from build123d import *

# Parameters (mm, degrees)
SKETCH_1_R          = 30
EXTRUDE_1_DEPTH     = 1
SKETCH_2_R          = 49
EXTRUDE_2_DEPTH     = 8
SKETCH_3_R          = 31
EXTRUDE_3_DEPTH     = 10
SKETCH_4_R          = 25
CUT_EXTRUDE_1_DEPTH = 1
SKETCH_5_R          = 15.5
CUT_EXTRUDE_2_DEPTH = 6
SKETCH_6_R          = 22
CUT_EXTRUDE_3_DEPTH = 6
SKETCH_7_R          = 15.5
CUT_EXTRUDE_4_DEPTH = 6
CHAMFER_1_SIZE2     = 6.5
CHAMFER_1_SIZE      = 0.798099646
CHAMFER_2_SIZE2     = 0.798099646
CHAMFER_2_SIZE      = 6.5
SKETCH_8_R          = 4.5
CUT_EXTRUDE_5_DEPTH = 10


with BuildPart() as part:
    # 草图1 → 凸台-拉伸1 (new body)
    with BuildSketch(Plane.XY):
        Circle(SKETCH_1_R)
    extrude(amount=EXTRUDE_1_DEPTH)

    # 草图2 → 凸台-拉伸2 (add)
    with BuildSketch(Plane.XY.offset(1)):
        Circle(SKETCH_2_R)
    extrude(amount=EXTRUDE_2_DEPTH)

    # 草图3 → 凸台-拉伸3 (add)
    with BuildSketch(Plane.XY.offset(9)):
        Circle(SKETCH_3_R)
    extrude(amount=EXTRUDE_3_DEPTH)

    # 草图4 → 切除-拉伸1 (cut)
    with BuildSketch(Plane.XY.offset(19)):
        Circle(SKETCH_4_R)
    extrude(amount=-CUT_EXTRUDE_1_DEPTH, mode=Mode.SUBTRACT)

    # 草图5 → 切除-拉伸2 (cut)
    with BuildSketch(Plane(origin=(0, 0, 0), x_dir=(-1, 0, 0), z_dir=(0, 0, -1))):
        Circle(SKETCH_5_R)
    extrude(amount=-CUT_EXTRUDE_2_DEPTH, mode=Mode.SUBTRACT)

    # 草图6 → 切除-拉伸3 (cut)
    with BuildSketch(Plane(origin=(0, 0, 6), x_dir=(-1, 0, 0), z_dir=(0, 0, -1))):
        Circle(SKETCH_6_R)
    extrude(amount=-CUT_EXTRUDE_3_DEPTH, mode=Mode.SUBTRACT)

    # 草图7 → 切除-拉伸4 (cut)
    with BuildSketch(Plane(origin=(0, 0, 12), x_dir=(-1, 0, 0), z_dir=(0, 0, -1))):
        Circle(SKETCH_7_R)
    extrude(amount=-CUT_EXTRUDE_4_DEPTH, mode=Mode.SUBTRACT)

    # 倒角1
    chamfer_1_edges = [part.edges().sort_by_distance(p)[0] for p in [
        (15.5, 0, 6),
    ]]
    chamfer_1_side = [part.faces().sort_by_distance(p)[0] for p in [
        (15.5, 0, 5.984038007),
    ]]
    chamfer(chamfer_1_edges, length=CHAMFER_1_SIZE - 0.0001, length2=CHAMFER_1_SIZE2 - 0.0001, reference=chamfer_1_side[0])  # a hair under: the kernel refuses the full size

    # 倒角2
    chamfer_2_edges = [part.edges().sort_by_distance(p)[0] for p in [
        (15.5, 0, 12),
    ]]
    chamfer_2_side = [part.faces().sort_by_distance(p)[0] for p in [
        (15.515961993, 0, 12),
    ]]
    chamfer(chamfer_2_edges, length=CHAMFER_2_SIZE - 0.0001, length2=CHAMFER_2_SIZE2 - 0.0001, reference=chamfer_2_side[0])  # a hair under: the kernel refuses the full size

    # 草图8 → 切除-拉伸5 (cut)
    with BuildSketch(Plane.XY.offset(9)):
        with Locations((0, 40)):
            Circle(SKETCH_8_R)
        with Locations((40, 0)):
            Circle(SKETCH_8_R)
        with Locations((0, -40)):
            Circle(SKETCH_8_R)
        with Locations((-40, 0)):
            Circle(SKETCH_8_R)
    extrude(amount=-CUT_EXTRUDE_5_DEPTH, mode=Mode.SUBTRACT)


solid = part.part
Work out the finished part from the listing and answer in its coordinate system (mm). A direction names the side the tool comes from. Round coordinates to 2 decimals unless told otherwise and drop trailing zeros. Order: outer loops, then holes, each group sorted by start corner. A loop starts at its lowest first (then second) coordinate and runs counter-clockwise, first axis right, second up. Notation, with made-up numbers: M 8.25,-32 L 64.25,-32 A16 ccw 64.25,-1 Z; hole C -19.5,20.25 d10. An arc over 180 degrees is marked long. Put each result on its own line as item: value. Start each with the question number.
Q1. Straight lines are drawn through the part: L1, parallel to Y at x = 0, z = 6.75; L2, parallel to Y at x = 0, z = 15.5; L3, parallel to Z at x = 22.5, y = -39. For each, find the intervals that lie inside material, in ascending order. Write a range as [from, to].
Q2. Flat-ended cylindrical pins translate along their axes: pin 1 (5 mm diameter, centred on x = -36.5, y = 31, fed in from +Z); pin 2 (22 mm diameter, centred on x = 10.5, y = -9, fed in from -Z); pin 3 (8 mm diameter, centred on x = 22.5, z = 5.5, fed in from +Y); pin 4 (4 mm diameter, centred on x = 38, z = 4.5, fed in from +Y). Find the tip coordinate at first contact, or state that the pin passes through.
Q3. Section A-A, the plane y = 40 is taken. Write down the section's boundary in (x, z).
Q4. A tool of negligible diameter and unlimited length cuts with its end or side. For faces 1 (the cylindrical face through (-29.97, 1.32, 0.49)), 2 (the cylindrical face through (4.769, -21.477, 8.958)), 3 (the cylindrical face through (-0.98, -44.39, 5.06)), 4 (the flat face through (-21, 14, 19)), 5 (the cylindrical face through (-4.036, 30.736, 13.93)), from which of +Z, -Z, +X, -X, +Y, -Y can it reach the whole face along a straight path? Write none if from no direction.
Q5. For a pull along Y with two mould halves and no side action, classify faces 6 (the cylindrical face through (26.34, 41.32, 4.94)), 7 (the conical face through (3.448, -15.528, 5.252)), 8 (the flat face through (13, -13, 0)), 9 (the cylindrical face through (-0.98, 35.61, 5.06)) as pulls with the +Y half, pulls with the -Y half, needs draft (parallel to the pull), parting line crosses it, or undercut.
Q6. Section C-C, the plane y = 0 is taken. Give the number of separate pieces and of enclosed holes in the cut face, and give its area (3 significant figures).
Findings below:
1. L1: y = [-49, -44.5], [-35.5, -22], [22, 35.5], [44.5, 49]
1. L2: y = [-31, -15.5], [15.5, 31]
1. L3: z = [1, 9]
2. pin 1: stops at z = 9
2. pin 2: stops at z = 0
2. pin 3: stops at y = 45.37
2. pin 4: stops at y = 33.24
3. outline: M -28.3,1 L -4.5,1 L -4.5,9 L -28.3,9 Z; M 4.5,1 L 28.3,1 L 28.3,9 L 4.5,9 Z
4. face 1: -Z
4. face 2: none
4. face 3: +Z, -Z
4. face 4: +Z, +X, -X, +Y, -Y
4. face 5: +Z
5. face 6: parting line crosses it
5. face 7: undercut
5. face 8: needs draft
5. face 9: undercut
6. separate pieces: 4
6. enclosed holes: 0
6. area: 624 mm^2
